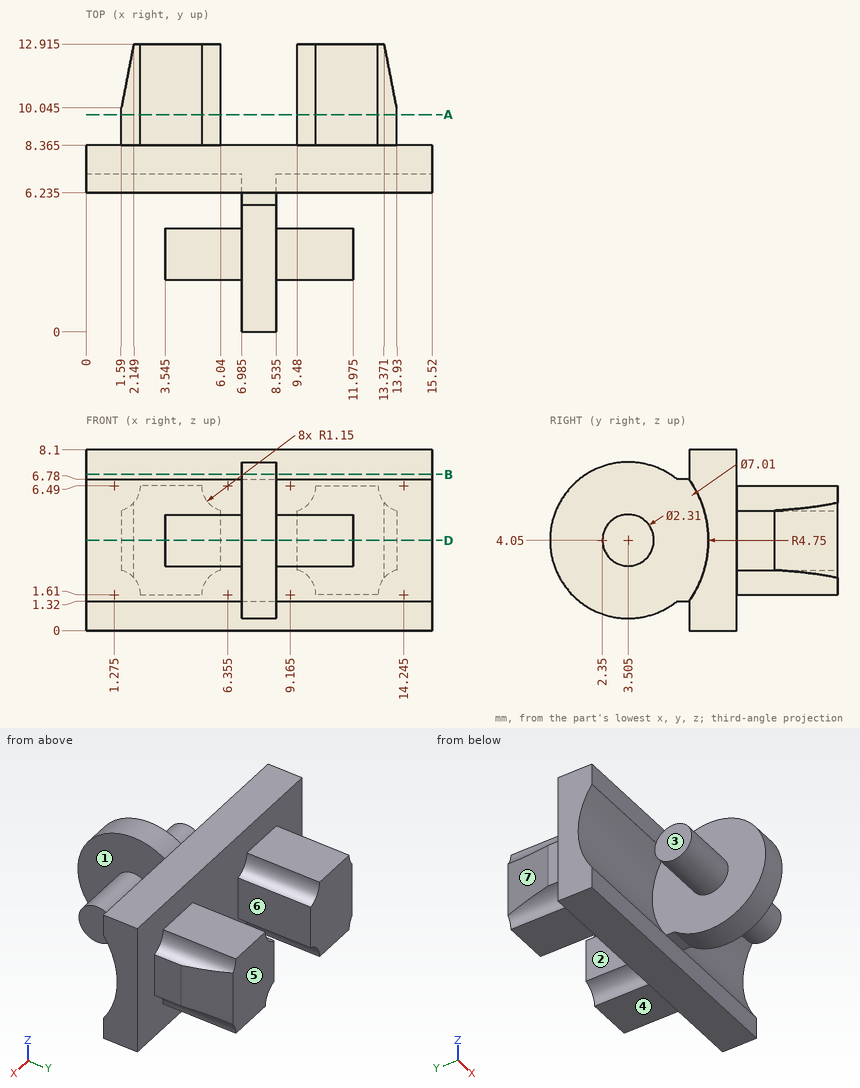
Here's the drawing with two shaded views (mm, measured from the low corner). I have some questions. A direction names the side the tool comes from. Give positions to 0.01 mm unless a question says otherwise; leave off trailing zeros. Order: outer loops, then holes, each group sorted by start corner. A loop starts at its lowest first (then second) coordinate and runs counter-clockwise, first axis right, second up. Notation, with made-up numbers: (26.25, 51.5) - (36.25, 51.5) arc R23 ccw to (36.25, 65.5) - close; hole circle Ø1 at (42, -33). An arc over 180 degrees is marked (long way). Use a Markdown table: item, result. Add a question column.
Q1. I'm going to push flat-ended pins straight in: pin 1 (3 mm diameter, centred on x = 11, y = 11.5, fed in from +Z); pin 2 (3 mm diameter, centred on x = 12, y = 11, fed in from -Z); pin 3 (0.5 mm diameter, centred on y = 9.5, z = 4.5, fed in from +X). Where does each tip first touch, or does it pass through?
Q2. If we section it at A-A on y = 9.75: Write out the boundary of the cut face in (x, z) (3 decimals), plus the area to 3 significant figures.
Q3. On a 3-axis mill with a long thin cutter (end or side, diameter ignored), from which of +Z, -Z, +X, -X, +Y, -Y can I reach the whole of each face in a straight line? I mean the marked faces 1, 2, 3 and 4. Say none if no direction works.
Q4. Please list where these lines run through material, in increasing order: line 1 along Y through (x, z) = (9.75, 7) (3 decimals); line 2 along X through (y, z) = (8.75, 5.25); line 3 along Y through (x, z) = (9, 4) (3 decimals).
Q5. If we section it at D-D on z = 4.05: Write out the boundary of the cut face in (x, y) (3 decimals), plus the area to 3 significant figures.
Q6. If we mould it in two halves opening along X, with no side actions, what happens to the marked faces 5, 6 and 7? For each: released by +X, released by -X, zero draft, split by the parting line, or undercut.
Q7. If we section it at B-B on z = 7: Write out the boundary of the cut face in (x, y) (3 decimals), plus the area to 3 significant figures.
Answers follow:
| question | item | result |
|---|---|---|
| 1 | pin 1 | stops at z = 6.49 |
| 1 | pin 2 | stops at z = 1.61 |
| 1 | pin 3 | stops at x = 13.93 |
| 2 | outline | (1.59, 2.716) arc R1.15 cw to (2.425, 1.61) - (5.205, 1.61) arc R1.15 cw to (6.04, 2.716) - (6.04, 5.384) arc R1.15 cw to (5.205, 6.49) - (2.425, 6.49) arc R1.15 cw to (1.59, 5.384) - close; (9.48, 2.716) arc R1.15 cw to (10.315, 1.61) - (13.095, 1.61) arc R1.15 cw to (13.93, 2.716) - (13.93, 5.384) arc R1.15 cw to (13.095, 6.49) - (10.315, 6.49) arc R1.15 cw to (9.48, 5.384) - close |
| 2 | area | 38.0 mm^2 |
| 3 | face 1 | +X |
| 3 | face 2 | +Z, -Z, +Y |
| 3 | face 3 | +Z, -Z, -X, -Y |
| 3 | face 4 | -Z, +X, -X, +Y |
| 4 | line 1 | y = 6.235 to 8.365 |
| 4 | line 2 | x = 1.59 to 6.04, 9.48 to 13.93 |
| 4 | line 3 | y = 2.351 to 4.659, 7.1 to 8.365 |
| 5 | outline | (0, 7.1) - (6.985, 7.1) - (6.985, 4.66) - (3.545, 4.66) - (3.545, 2.35) - (6.985, 2.35) - (6.985, 0) - (8.535, 0) - (8.535, 2.35) - (11.975, 2.35) - (11.975, 4.66) - (8.535, 4.66) - (8.535, 7.1) - (15.52, 7.1) - (15.52, 8.365) - (13.93, 8.365) - (13.93, 10.045) - (13.371, 12.915) - (9.48, 12.915) - (9.48, 8.365) - (6.04, 8.365) - (6.04, 12.915) - (2.149, 12.915) - (1.59, 10.045) - (1.59, 8.365) - (0, 8.365) - close |
| 5 | area | 85.4 mm^2 |
| 6 | face 5 | zero draft |
| 6 | face 6 | undercut |
| 6 | face 7 | released by -X |
| 7 | outline | (0, 6.235) - (15.52, 6.235) - (15.52, 8.365) - (0, 8.365) - close; (6.985, 1.612) - (8.535, 1.612) - (8.535, 5.398) - (6.985, 5.398) - close |
| 7 | area | 38.9 mm^2 |
